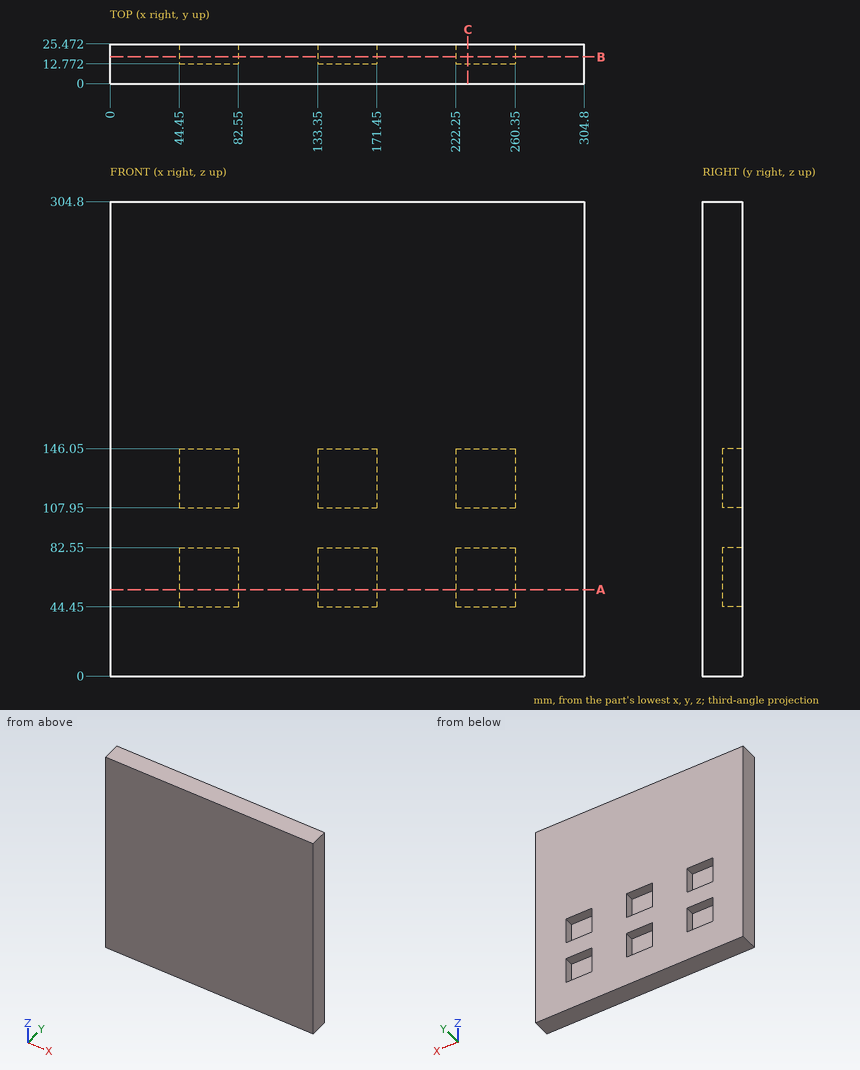
For this review, use the dimensioned drawing (mm, ordinates from the lowest corner) and the shaded views. Round coordinates to 2 decimals unless told otherwise and drop trailing zeros. Write each loop counter-clockwise with the first axis right and the second up, starting at its lowest first coordinate (ties: lowest second). Pieces come first, ordered by that corner, then holes. Notation, with made-up numbers: (26.25, 85) - (50.25, 85) arc R10 ccw to (50.25, 93) - close; hole circle Ø3 at (86, 34). An arc over 180 degrees is marked (long way). Use a Markdown table: item, result.
Q1. We need section C-C (x = 230). Give the boundary of the cut face in (y, z), plus the area to 3 significant figures.
Derived:
| item | result |
|---|---|
| outline | (0, 0) - (25.47, 0) - (25.47, 44.45) - (12.77, 44.45) - (12.77, 82.55) - (25.47, 82.55) - (25.47, 107.95) - (12.77, 107.95) - (12.77, 146.05) - (25.47, 146.05) - (25.47, 304.8) - (0, 304.8) - close |
| area | 6,800 mm2 |
Q2. Clearance check with a flat-ended pin moving along its axis: pin 1 (19 mm diameter, centred on x = 61, z = 126.5, fed in from +Y). State where the tip first meets the part, or that it passes through.
Derived:
| item | result |
|---|---|
| pin 1 | stops at y = 12.77 |
Q3. Wall thickness on line 1 along Z through (x, y) = (67.5, 18.25); line 2 along X through (y, z) = (14.75, 121): over which ranges is each line inside the solid? List them lowest first.
Derived:
| item | result |
|---|---|
| line 1 | z = 0 to 44.45, 82.55 to 107.95, 146.05 to 304.8 |
| line 2 | x = 0 to 44.45, 82.55 to 133.35, 171.45 to 222.25, 260.35 to 304.8 |
Q4. We need section B-B (y = 17.25). Give the boundary of the cut face in (x, z), plus the area to 3 significant figures.
Derived:
| item | result |
|---|---|
| outline | (0, 0) - (304.8, 0) - (304.8, 304.8) - (0, 304.8) - close; hole (44.45, 44.45) - (82.55, 44.45) - (82.55, 82.55) - (44.45, 82.55) - close; hole (44.45, 107.95) - (82.55, 107.95) - (82.55, 146.05) - (44.45, 146.05) - close; hole (133.35, 44.45) - (171.45, 44.45) - (171.45, 82.55) - (133.35, 82.55) - close; hole (133.35, 107.95) - (171.45, 107.95) - (171.45, 146.05) - (133.35, 146.05) - close; hole (222.25, 44.45) - (260.35, 44.45) - (260.35, 82.55) - (222.25, 82.55) - close; hole (222.25, 107.95) - (260.35, 107.95) - (260.35, 146.05) - (222.25, 146.05) - close |
| area | 84,200 mm2 |
Q5. We need section A-A (z = 55.5). Give the boundary of the cut face in (x, y).
Derived:
| item | result |
|---|---|
| outline | (0, 0) - (304.8, 0) - (304.8, 25.47) - (260.35, 25.47) - (260.35, 12.77) - (222.25, 12.77) - (222.25, 25.47) - (171.45, 25.47) - (171.45, 12.77) - (133.35, 12.77) - (133.35, 25.47) - (82.55, 25.47) - (82.55, 12.77) - (44.45, 12.77) - (44.45, 25.47) - (0, 25.47) - close |
